```python
from build123d import *

# Parameters (mm, degrees)
BOSS_EXTRUDE4_DEPTH = 21
BOSS_EXTRUDE5_START = 3.5
BOSS_EXTRUDE5_DEPTH = 3.5
SKETCH4_W           = 27
SKETCH4_H           = 19
CUT_EXTRUDE4_DEPTH  = 72.268857154
SKETCH3_5_W         = 24.4
SKETCH3_5_H         = 12.66
BOSS_EXTRUDE6_DEPTH = 2
SKETCH5_W           = 51
SKETCH5_H           = 29
BOSS_EXTRUDE7_DEPTH = 10
CUT_EXTRUDE5_DEPTH  = 75.828136419
CUT_EXTRUDE6_REACH  = 76.828
SKETCH8_W           = 24.5
SKETCH8_H           = 19.5
CHAMFER1_SIZE       = 2


with BuildPart() as part:
    # Sketch3 → Boss-Extrude4 (new body)
    with BuildSketch(Plane(origin=(0, 0, 0), x_dir=(1, 0, 0), z_dir=(0, 1, 0))):
        with BuildLine():
            Line((-27, 15), (-27, -39.5))
            ThreePointArc((-27, -39.5), (-26.414213562, -40.914213562), (-25, -41.5))
            Line((-25, -41.5), (25, -41.5))
            ThreePointArc((25, -41.5), (26.414213562, -40.914213562), (27, -39.5))
            Line((27, -39.5), (27, 15))
            ThreePointArc((27, 15), (26.414213562, 16.414213562), (25, 17))
            Line((25, 17), (-25, 17))
            ThreePointArc((-25, 17), (-26.414213562, 16.414213562), (-27, 15))
        make_face()
    extrude(amount=-BOSS_EXTRUDE4_DEPTH)

    # Sketch3<3> → Boss-Extrude5 (add)
    with BuildSketch(Plane(origin=(0, 0, 0), x_dir=(1, 0, 0), z_dir=(0, 1, 0)).offset(BOSS_EXTRUDE5_START)):
        with BuildLine():
            Line((-27, 15), (-27, -39.5))
            ThreePointArc((-27, -39.5), (-26.414213562, -40.914213562), (-25, -41.5))
            Line((-25, -41.5), (25, -41.5))
            ThreePointArc((25, -41.5), (26.414213562, -40.914213562), (27, -39.5))
            Line((27, -39.5), (27, 15))
            ThreePointArc((27, 15), (26.414213562, 16.414213562), (25, 17))
            Line((25, 17), (-25, 17))
            ThreePointArc((-25, 17), (-26.414213562, 16.414213562), (-27, 15))
        make_face()
        Polygon((0, 12), (-1.1, 12), (-1.1, -3.66), (-25.5, -3.66), (-25.5, 15.5), (25.5, 15.5), (25.5, -0.96), (0, -0.96), align=None, mode=Mode.SUBTRACT)
    extrude(amount=-BOSS_EXTRUDE5_DEPTH)

    # Sketch4 → Cut-Extrude4 (cut, through all)
    with BuildSketch(Plane.ZY.offset(27)):
        with Locations((-1.5, -9.5)):
            Rectangle(SKETCH4_W, SKETCH4_H)
    extrude(amount=-CUT_EXTRUDE4_DEPTH, mode=Mode.SUBTRACT)

    # Sketch3<5> → Boss-Extrude6 (add)
    with BuildSketch(Plane(origin=(0, 0, 0), x_dir=(1, 0, 0), z_dir=(0, 1, 0))):
        with Locations((-13.3, 5.67)):
            Rectangle(SKETCH3_5_W, SKETCH3_5_H)
        Polygon((25.5, 12), (0, 12), (0, -0.96), (25.5, -0.96), (25.5, -0.5), align=None)
    extrude(amount=BOSS_EXTRUDE6_DEPTH)

    # Sketch5 → Boss-Extrude7 (add)
    # profile 1 of 2: a face of its own
    with BuildSketch(Plane.XZ.offset(21)):
        with BuildLine():
            ThreePointArc((25, -17), (26.414213562, -16.414213562), (27, -15))
            Line((27, -15), (27, 39.5))
            ThreePointArc((27, 39.5), (26.414213562, 40.914213562), (25, 41.5))
            Line((25, 41.5), (-25, 41.5))
            ThreePointArc((-25, 41.5), (-26.414213562, 40.914213562), (-27, 39.5))
            Line((-27, 39.5), (-27, -15))
            ThreePointArc((-27, -15), (-26.414213562, -16.414213562), (-25, -17))
            Line((-25, -17), (25, -17))
        make_face()
        with Locations((0, -1)):
            Rectangle(SKETCH5_W, SKETCH5_H, mode=Mode.SUBTRACT)
    # profile 2 of 2: a face of its own
    with BuildSketch(Plane.XZ.offset(21)):
        with BuildLine():
            ThreePointArc((25, -17), (26.414213562, -16.414213562), (27, -15))
            Line((27, -15), (27, 39.5))
            ThreePointArc((27, 39.5), (26.414213562, 40.914213562), (25, 41.5))
            Line((25, 41.5), (-25, 41.5))
            ThreePointArc((-25, 41.5), (-26.414213562, 40.914213562), (-27, 39.5))
            Line((-27, 39.5), (-27, -15))
            ThreePointArc((-27, -15), (-26.414213562, -16.414213562), (-25, -17))
            Line((-25, -17), (25, -17))
        make_face()
        with Locations((0, -1)):
            Rectangle(SKETCH5_W, SKETCH5_H, mode=Mode.SUBTRACT)
    extrude(amount=BOSS_EXTRUDE7_DEPTH)

    # Sketch6 → Cut-Extrude5 (cut, through all)
    with BuildSketch(Plane.ZY.offset(27)):
        with BuildLine():
            Line((-10.438825699, -23), (8.061174301, -23))
            ThreePointArc((8.061174301, -23), (8.768281082, -23.292893219), (9.061174301, -24))
            Line((9.061174301, -24), (9.061174301, -27))
            ThreePointArc((9.061174301, -27), (8.768281082, -27.707106781), (8.061174301, -28))
            Line((8.061174301, -28), (-10.438825699, -28))
            ThreePointArc((-10.438825699, -28), (-11.14593248, -27.707106781), (-11.438825699, -27))
            Line((-11.438825699, -27), (-11.438825699, -24))
            ThreePointArc((-11.438825699, -24), (-11.14593248, -23.292893219), (-10.438825699, -23))
        make_face()
    extrude(amount=-CUT_EXTRUDE5_DEPTH, mode=Mode.SUBTRACT)

    # Sketch8 → Cut-Extrude6 (cut, up to next)
    with BuildSketch(Plane(origin=(27, 0, 0), x_dir=(0, 0, -1), z_dir=(1, 0, 0)), mode=Mode.PRIVATE) as cut_extrude6_sk1:
        with Locations((-27.25, -9.75)):
            Rectangle(SKETCH8_W, SKETCH8_H)
    cut_extrude6_tool1 = extrude(cut_extrude6_sk1.sketch, amount=-CUT_EXTRUDE6_REACH, mode=Mode.PRIVATE) & part.part
    add(cut_extrude6_tool1.solids().sort_by_distance((27, -9.75, 27.25))[0], mode=Mode.SUBTRACT)

    # Chamfer1
    chamfer1_edges = [part.edges().sort_by_distance(p)[0] for p in [
        (25.5, -26, -15.5),
        (-25.5, -21, -1),
        (-25.5, -26, -15.5),
        (0, -21, 13.5),
        (-25.5, -26, 13.5),
        (25.5, -26, 13.5),
        (0, -21, -15.5),
        (25.5, -21, -1),
        (0, 0, 12),
        (0, -19, 12),
    ]]
    chamfer(chamfer1_edges, length=CHAMFER1_SIZE - 0.0001)  # a hair under: the kernel refuses the full size


solid = part.part
```
Input: part model. Units: mm. Frame: model coordinates. A direction names the side the tool comes from. Round coordinates to 2 decimals unless told otherwise and drop trailing zeros. Order: outer loops, then holes, each group sorted by start corner. A loop starts at its lowest first (then second) coordinate and runs counter-clockwise, first axis right, second up. Notation, with made-up numbers: (24.25, 43) - (52.25, 43) arc R32 ccw to (52.25, 73) - close; hole circle Ø11 at (2.25, 56.25). An arc over 180 degrees is marked (long way). Answer in a Markdown table with one row per item.
Item 1: Reachability of faces 5 (the flat face through (0, 3.5, 18)), 6 (the flat face through (-25.5, -29, -1)), 7 (the flat face through (0, -19, -3)), 8 (the flat face through (0, 1, -12)), 9 (the cylindrical face through (-26.43, -13.51, -16.4)) from +Z, -Z, +X, -X, +Y, -Y: full face, straight path, thin tool, end or side. Return the list, or none.
Model answer:
| item | result |
|---|---|
| face 5 | +Z, -Z, +X, -X, +Y |
| face 6 | -Y |
| face 7 | +X, -X |
| face 8 | +Y |
| face 9 | -Z, -X, +Y, -Y |
Item 2: Section query A-A (z = -0.5). Give the number of separate pieces and of enclosed holes in the cut face, then the cut area to 3 significant figures.
Model answer:
| item | result |
|---|---|
| separate pieces | 4 |
| enclosed holes | 0 |
| area | 241 mm² |
Item 3: Pin query (flat end, axial travel): pin 1 (0.6 mm diameter, centred on x = 2.5, z = -15, fed in from +Y); pin 2 (12.5 mm diameter, centred on x = 6.5, z = 0.5, fed in from +Y); pin 3 (8 mm diameter, centred on x = -13.5, z = -2.5, fed in from -Y); pin 4 (12.5 mm diameter, centred on x = -6.5, z = -7.5, fed in from -Y). Return the tip coordinate at first contact, or that it passes through.
Model answer:
| item | result |
|---|---|
| pin 1 | stops at y = 0 |
| pin 2 | stops at y = 3.5 |
| pin 3 | stops at y = -21 |
| pin 4 | stops at y = -21.25 |
Item 4: Mould query, pull axis X, two halves, no side actions, for faces 1 (the flat face through (-26, -26, -11.439)), 2 (the cylindrical face through (26.43, -13.51, 40.9)), 3 (the flat face through (-27, -17, 13)), 4 (the flat face through (13, 2, -6)). Classes: released by +X, released by -X, zero draft, split by the parting line, or undercut.
Model answer:
| item | result |
|---|---|
| face 1 | zero draft |
| face 2 | released by +X |
| face 3 | released by -X |
| face 4 | undercut |
Item 5: Section query D-D (x = 11). Return the cut outline in (y, z), then the cut area to 3 significant figures.
Model answer:
| item | result |
|---|---|
| outline | (-31, -17) - (3.5, -17) - (3.5, -15.5) - (0, -15.5) - (0, -15) - (-19, -15) - (-19, 10) - (-17, 12) - (-2, 12) - (0, 10) - (0, -12) - (2, -12) - (2, 0.96) - (3.5, 0.96) - (3.5, 41.5) - (-31, 41.5) - (-31, 13.5) - (-23, 13.5) - (-21, 11.5) - (-21, -13.5) - (-23, -15.5) - (-31, -15.5) - close; hole (-19.5, 15) - (0, 15) - (0, 39.5) - (-19.5, 39.5) - close |
| area | 714 mm² |
Item 6: Line query: line 1 (Z direction, x = -19.5, y = -15); line 2 (Y direction, x = 10.5, z = -1); line 3 (Z direction, x = 11, y = -26.5). Output: solid intervals per line, ascending.
Model answer:
| item | result |
|---|---|
| line 1 | z = -17 to -15, 12 to 15, 39.5 to 41.5 |
| line 2 | y = -21 to -19, 0 to 2 |
| line 3 | z = -17 to -15.5, 13.5 to 41.5 |
Item 7: Section query B-B (x = -9). Return the cut outline in (y, z).
Model answer:
| item | result |
|---|---|
| outline | (-31, -17) - (3.5, -17) - (3.5, -15.5) - (0, -15.5) - (0, -15) - (-19, -15) - (-19, 10) - (-17, 12) - (-2, 12) - (0, 10) - (0, 3.66) - (3.5, 3.66) - (3.5, 41.5) - (-31, 41.5) - (-31, 13.5) - (-23, 13.5) - (-21, 11.5) - (-21, -13.5) - (-23, -15.5) - (-31, -15.5) - close; (0, -12) - (2, -12) - (2, 0.66) - (0, 0.66) - close; hole (-19.5, 15) - (0, 15) - (0, 39.5) - (-19.5, 39.5) - close |
Item 8: Section query C-C (y = -9). Return the cut outline in (x, z).
Model answer:
| item | result |
|---|---|
| outline | (-27, -15) arc R2 ccw to (-25, -17) - (25, -17) arc R2 ccw to (27, -15) - close; (-27, 12) - (27, 12) - (27, 15) - (-27, 15) - close; (-27, 39.5) - (27, 39.5) arc R2 ccw to (25, 41.5) - (-25, 41.5) arc R2 ccw to start |
